```python
from build123d import *

# Parameters (mm, degrees)
F0_W           = 129.58
F0_H           = 66
F1_DEPTH       = 22
F3_D           = 3
F3_CBORE_D     = 5.5
F3_CBORE_DEPTH = 2.4
F4_T           = 2.54
F5_R           = 1


# Not quite as in the source:
# - a shell that OpenCascade refuses in one call is made with other operations: the cavity is built on its own and cut out


with BuildPart() as f1:
    # F0 (on Front) → F1 (new body)
    with BuildSketch(Plane.XZ):
        with Locations((64.79, 33)):
            Rectangle(F0_W, F0_H)
    extrude(amount=F1_DEPTH)

    # F3 (through all)
    with Locations(Plane.XZ.offset(22)):
        with Locations((4, 62), (4, 4), (125.58, 4), (125.58, 62)):
            CounterBoreHole(F3_D / 2, F3_CBORE_D / 2, F3_CBORE_DEPTH)

    # F4: shell of thickness 2.54, made by hand


with BuildPart() as f4_core1:
    # F4_t2: copy of F1
    add(f1.part)

    # the walls: a layer under each face that stays
    f4_faces = [f4_core1.faces().sort_by_distance(p)[0] for p in [
        (0, -11, 33),
        (64.79, -11, 66),
        (64.79, -11, 0),
        (64.79, -22, 33),
        (129.58, -11, 33),
        (2.5, -9.8, 4),
        (124.08, -9.8, 4),
        (2.5, -9.8, 62),
        (124.08, -9.8, 62),
        (1.25, -20.8, 4),
        (122.83, -20.8, 4),
        (1.25, -20.8, 62),
        (122.83, -20.8, 62),
        (2.1666666667, -19.6, 2.1666666667),
        (123.7466666667, -19.6, 2.1666666667),
        (2.1666666667, -19.6, 60.1666666667),
        (123.7466666667, -19.6, 60.1666666667),
    ]]
    thicken(f4_faces, amount=-F4_T, mode=Mode.SUBTRACT)

    # F4_s3 → F4_t4 (revolve, cut)
    with BuildSketch(Plane.XY.offset(4)):
        Polygon((6.7246, -19.6254), (9.29, -19.6), (9.29, -17.06), (6.75, -17.06), align=None)
    revolve(axis=Axis((4, -19.6, 4), (0, -1, 0)), mode=Mode.SUBTRACT)

    # F4_s5 → F4_t6 (revolve, cut)
    with BuildSketch(Plane.XY.offset(4)):
        Polygon((128.3046, -19.6254), (130.87, -19.6), (130.87, -17.06), (128.33, -17.06), align=None)
    revolve(axis=Axis((125.58, -19.6, 4), (0, -1, 0)), mode=Mode.SUBTRACT)

    # F4_s7 → F4_t8 (revolve, cut)
    with BuildSketch(Plane.XY.offset(62)):
        Polygon((6.7246, -19.6254), (9.29, -19.6), (9.29, -17.06), (6.75, -17.06), align=None)
    revolve(axis=Axis((4, -19.6, 62), (0, -1, 0)), mode=Mode.SUBTRACT)

    # F4_s9 → F4_t10 (revolve, cut)
    with BuildSketch(Plane.XY.offset(62)):
        Polygon((128.3046, -19.6254), (130.87, -19.6), (130.87, -17.06), (128.33, -17.06), align=None)
    revolve(axis=Axis((125.58, -19.6, 62), (0, -1, 0)), mode=Mode.SUBTRACT)


with BuildPart() as f1_1:
    add(f1.part)

    # what is left inside the walls is the cavity
    f4_cavity = [f4_core1.part.solids().sort_by_distance(p)[0] for p in [
        (64.79, -0.0254, 22.846667),
    ]]
    add(f4_cavity, mode=Mode.SUBTRACT)

    # F5
    f5_edges = [f1_1.edges().sort_by_distance(p)[0] for p in [
        (64.79, -22, 66),
        (0, -11, 66),
        (0, -11, 0),
        (129.58, -11, 66),
        (129.58, -11, 0),
        (64.79, -22, 0),
        (129.58, -22, 33),
        (0, -22, 33),
    ]]
    fillet(f5_edges, radius=F5_R)


solid = f1_1.part
```
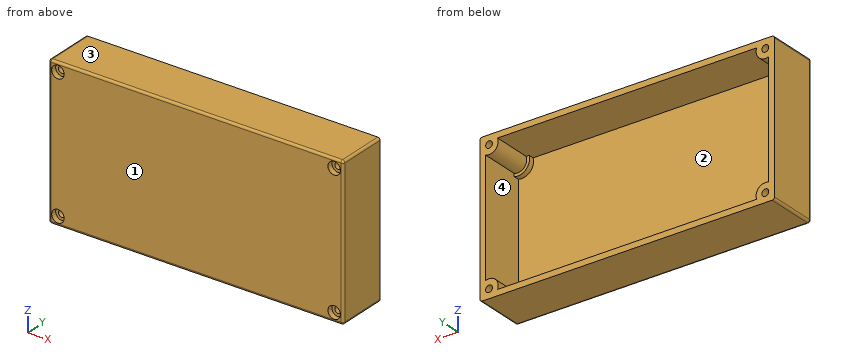
Input: part model. Units: mm. Frame: model coordinates. Face numbers are marked on the shaded views. Round coordinates to 2 decimals unless told otherwise and drop trailing zeros. Loops run counter-clockwise (first coordinate to the right, second up) from the corner with the lowest first, then second, coordinate; pieces in that order, holes last. Notation, with made-up numbers: (33.5, 86) -> (38.5, 86) arc R10 ccw to (38.5, 98) -> close; hole circle Ø1 at (8, 43). An arc over 180 degrees is marked (long way). One line per item, written item: value.
(1) Section A-A (z = 62). Give the number of separate pieces and of enclosed holes in the cut face, plus the area to 3 significant figures.
Geometry check:
separate pieces: 3
enclosed holes: 0
area: 504 mm2
(2) Section C-C (y = -7.5). Return the cut outline in (x, z), plus the area to 3 significant figures.
Geometry check:
outline: (0, 1) arc R1 ccw to (1, 0) -> (128.58, 0) arc R1 ccw to (129.58, 1) -> (129.58, 65) arc R1 ccw to (128.58, 66) -> (1, 66) arc R1 ccw to (0, 65) -> close; hole circle Ø3 at (4, 4); hole circle Ø3 at (4, 62); hole (2.54, 7.77) arc R4.04 cw to (7.77, 2.54) -> (121.81, 2.54) arc R4.04 cw to (127.04, 7.77) -> (127.04, 58.23) arc R4.04 cw to (121.81, 63.46) -> (7.77, 63.46) arc R4.04 cw to (2.54, 58.23) -> close; hole circle Ø3 at (125.58, 4); hole circle Ø3 at (125.58, 62)
area: 1,040 mm2
(3) Mould query, pull axis Z, two halves, no side actions, for the marked faces 1, 2, 3 and 4. Classes: pulls with the +Z half, pulls with the -Z half, needs draft (parallel to the pull), parting line crosses it, or undercut.
Geometry check:
face 1: needs draft
face 2: undercut
face 3: pulls with the +Z half
face 4: undercut
(4) Section D-D (z = 39.5). Return the cut outline in (x, y).
Geometry check:
outline: (0, -21) arc R1 ccw to (1, -22) -> (128.58, -22) arc R1 ccw to (129.58, -21) -> (129.58, 0) -> (127.04, 0) -> (127.04, -19.46) -> (2.54, -19.46) -> (2.54, 0) -> (0, 0) -> close
(5) Material intervals for line 1 (Z direction, x = 125.58, y = -20.05); line 2 (X direction, y = -3.5, z = 15); line 3 (Z direction, x = 16, y = -18), sorted ascending. Write a range as [from, to].
Geometry check:
line 1: [0, 1.25], [6.75, 59.25], [64.75, 66]
line 2: [0, 2.54], [127.04, 129.58]
line 3: [0, 2.54], [63.46, 66]
(6) Pin query (flat end, axial travel): pin 1 (4 mm diameter, centred on x = 125.58, z = 4, fed in from -Y); pin 2 (1.8 mm diameter, centred on x = 4, z = 62, fed in from +Y). Return the tip coordinate at first contact, or that it passes through.
Geometry check:
pin 1: y = -19.6
pin 2: through
